from build123d import *

# Parameters (mm, degrees)
SKETCH1_W           = 131
SKETCH1_H           = 98
SKETCH1_W_2         = 125
SKETCH1_H_2         = 90
BOSS_EXTRUDE1_DEPTH = 80
SKETCH2_W           = 131
SKETCH2_H           = 98
BOSS_EXTRUDE2_DEPTH = 3
SKETCH4_W           = 125
SKETCH4_H           = 90
SKETCH4_W_2         = 119.5
SKETCH4_H_2         = 84.5
BOSS_EXTRUDE3_DEPTH = 3
SKETCH5_W           = 15
SKETCH5_H           = 73
CUT_EXTRUDE1_DEPTH  = 143.457888514
CUT_EXTRUDE2_REACH  = 141.736
SKETCH6_W           = 20
SKETCH6_H           = 57
CUT_EXTRUDE3_REACH  = 141.736
SKETCH7_W           = 15
SKETCH7_H           = 20
SKETCH8_W           = 5
SKETCH8_H           = 10
BOSS_EXTRUDE4_DEPTH = 10


with BuildPart() as part:
    # Sketch1 → Boss-Extrude1 (new body)
    with BuildSketch(Plane(origin=(0, 0, 0), x_dir=(1, 0, 0), z_dir=(0, 1, 0))):
        Rectangle(SKETCH1_W, SKETCH1_H)
        Rectangle(SKETCH1_W_2, SKETCH1_H_2, mode=Mode.SUBTRACT)
    extrude(amount=BOSS_EXTRUDE1_DEPTH)

    # Sketch2 → Boss-Extrude2 (add)
    with BuildSketch(Plane.XZ):
        Rectangle(SKETCH2_W, SKETCH2_H)
    extrude(amount=BOSS_EXTRUDE2_DEPTH)

    # Sketch4 → Boss-Extrude3 (add)
    with BuildSketch(Plane(origin=(0, 0, 0), x_dir=(1, 0, 0), z_dir=(0, 1, 0))):
        Rectangle(SKETCH4_W, SKETCH4_H)
        with Locations((-0.25, 0.25)):
            Rectangle(SKETCH4_W_2, SKETCH4_H_2, mode=Mode.SUBTRACT)
    extrude(amount=BOSS_EXTRUDE3_DEPTH)

    # Sketch5 → Cut-Extrude1 (cut, through all)
    with BuildSketch(Plane(origin=(0, 0, -49), x_dir=(-1, 0, 0), z_dir=(0, 0, -1))):
        with Locations((22.5, 43.5)):
            Rectangle(SKETCH5_W, SKETCH5_H)
    extrude(amount=-CUT_EXTRUDE1_DEPTH, mode=Mode.SUBTRACT)

    # Sketch6 → Cut-Extrude2 (cut, up to next)
    with BuildSketch(Plane(origin=(0, 0, 45), x_dir=(-1, 0, 0), z_dir=(0, 0, -1)), mode=Mode.PRIVATE) as cut_extrude2_sk1:
        with Locations((-37.5, 51.5)):
            Rectangle(SKETCH6_W, SKETCH6_H)
    cut_extrude2_tool1 = extrude(cut_extrude2_sk1.sketch, amount=-CUT_EXTRUDE2_REACH, mode=Mode.PRIVATE) & part.part
    add(cut_extrude2_tool1.solids().sort_by_distance((37.5, 51.5, 45))[0], mode=Mode.SUBTRACT)

    # Sketch7 → Cut-Extrude3 (cut, up to next)
    with BuildSketch(Plane.XY.offset(-45), mode=Mode.PRIVATE) as cut_extrude3_sk1:
        with Locations((40, 70)):
            Rectangle(SKETCH7_W, SKETCH7_H)
    cut_extrude3_tool1 = extrude(cut_extrude3_sk1.sketch, amount=-CUT_EXTRUDE3_REACH, mode=Mode.PRIVATE) & part.part
    # Sketch7 → Cut-Extrude3 (cut, up to next)
    with BuildSketch(Plane.XY.offset(-45), mode=Mode.PRIVATE) as cut_extrude3_sk2:
        with Locations((7.5, 70)):
            Rectangle(SKETCH7_W, SKETCH7_H)
    cut_extrude3_tool2 = extrude(cut_extrude3_sk2.sketch, amount=-CUT_EXTRUDE3_REACH, mode=Mode.PRIVATE) & part.part
    add(cut_extrude3_tool1.solids().sort_by_distance((40, 70, -45))[0], mode=Mode.SUBTRACT)
    add(cut_extrude3_tool2.solids().sort_by_distance((7.5, 70, -45))[0], mode=Mode.SUBTRACT)

    # Sketch8 → Boss-Extrude4 (add)
    with BuildSketch(Plane.XY.offset(-45)):
        with Locations((-2.5, 75)):
            Rectangle(SKETCH8_W, SKETCH8_H)
        with Locations((17.5, 75)):
            Rectangle(SKETCH8_W, SKETCH8_H)
        with Locations((30, 75)):
            Rectangle(SKETCH8_W, SKETCH8_H)
        with Locations((50, 75)):
            Rectangle(SKETCH8_W, SKETCH8_H)
    extrude(amount=BOSS_EXTRUDE4_DEPTH)


solid = part.part
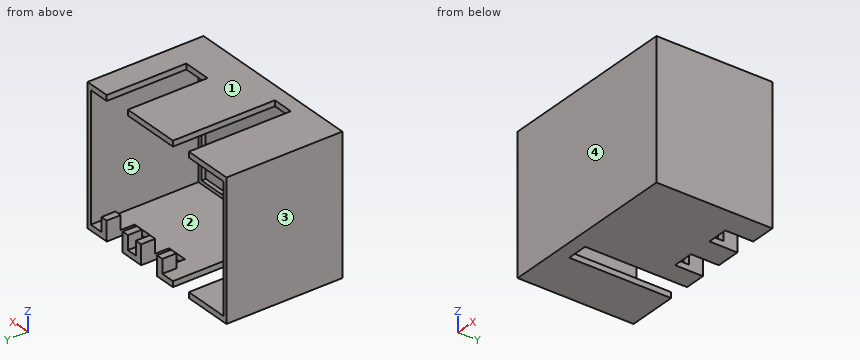
CAD build for the part. Positions are in the model's coordinates, mm. Face numbers are marked on the shaded views. A direction names the side the tool comes from. Round coordinates to 2 decimals unless told otherwise and drop trailing zeros. Loops run counter-clockwise (first coordinate to the right, second up) from the corner with the lowest first, then second, coordinate; pieces in that order, holes last. Notation, with made-up numbers: M -31.75,34 L 1.25,34 A29 cw 1.25,66 Z; hole C 13,-36.75 d2. An arc over 180 degrees is marked long. One line per question, with ' | ' between items. Start each with the question number.
Item 1: Cut at C-C, the plane z = -37. Write the cut outline in (x, y), plus the area to 3 significant figures.
Item 2: Which spindle directions (+Z, -Z, +X, -X, +Y, -Y) get a long thin tool onto all of the face, cutting with end or side? Do the marked faces 4 and 5. Say none if no direction does.
Item 3: Cut at B-B, the plane y = 66. Write the cut outline in (x, z).
Item 4: Two-plate mould, pull along Z, no slides. Class the marked faces 1, 2 and 3: pulls with the +Z half, pulls with the -Z half, needs draft (parallel to the pull), parting line crosses it, or undercut.
Item 5: Pin check, flat tips, straight feed: pin 1 Ø2 at (x, z) = (40.5, 47.5) entering from +Y; pin 2 Ø4.5 at (x, z) = (43.5, -46.5) entering from +Y; pin 3 Ø1.2 at (x, z) = (-23.5, 47) entering from +Y. Stop position of each tip, or through.
Item 6: Cut at A-A, the plane y = 19. Write the cut outline in (x, z).
Item 7: Cut at D-D, the plane x = 5.5. Write the cut outline in (y, z).
Item 8: Wall check: line 1 (X direction, y = 75.5, z = -40); line 2 (Z direction, x = -10.5, y = 48); line 3 (X direction, y = 29, z = 11). Give the ranges that are in metal, low to high.
Responses:
1) outline: M -65.5,-3 L 65.5,-3 L 65.5,80 L 62.5,80 L 62.5,3 L 59.5,3 L 59.5,0 L -60,0 L -60,3 L -62.5,3 L -62.5,80 L -65.5,80 Z; M -5,70 L 0,70 L 0,80 L -5,80 Z; M 15,70 L 20,70 L 20,80 L 15,80 Z; M 27.5,70 L 32.5,70 L 32.5,80 L 27.5,80 Z; M 47.5,70 L 52.5,70 L 52.5,80 L 47.5,80 Z | area: 1,090 mm²
2) face 4: +Z, -Z, +X, -X, -Y | face 5: +Y
3) outline: M -65.5,-49 L -30,-49 L -30,-45 L -62.5,-45 L -62.5,45 L -30,45 L -30,49 L -65.5,49 Z; M -15,-49 L 0,-49 L 0,-45 L -15,-45 Z; M -15,45 L 27.5,45 L 27.5,49 L -15,49 Z; M 15,-49 L 32.5,-49 L 32.5,-45 L 15,-45 Z; M 47.5,-49 L 65.5,-49 L 65.5,49 L 47.5,49 L 47.5,45 L 62.5,45 L 62.5,-45 L 47.5,-45 Z
4) face 1: pulls with the +Z half | face 2: undercut | face 3: needs draft
5) pin 1: stops at y = 23 | pin 2: stops at y = 60 | pin 3: stops at y = 7
6) outline: M -65.5,-49 L -30,-49 L -30,-45 L -62.5,-45 L -62.5,45 L -30,45 L -30,49 L -65.5,49 Z; M -15,-49 L 65.5,-49 L 65.5,49 L -15,49 L -15,45 L 62.5,45 L 62.5,-45 L -15,-45 Z
7) outline: M -3,-49 L 60,-49 L 60,-45 L 3,-45 L 3,-42.5 L 0,-42.5 L 0,42 L 3,42 L 3,45 L 80,45 L 80,49 L -3,49 Z
8) line 1: x = -65.5 to -62.5, -5 to 0, 15 to 20, 27.5 to 32.5, 47.5 to 52.5, 62.5 to 65.5 | line 2: z = -49 to -45, 45 to 49 | line 3: x = -65.5 to -62.5, 62.5 to 65.5
